Autodesk Inventor part; units mm, degrees
ref_plane "YZ Plane" through (0, 0, 0) normal (1, 0, 0) x (0, 1, 0)
ref_plane "XZ Plane" through (0, 0, 0) normal (0, 1, 0) x (-1, 0, 0)
ref_plane "XY Plane" through (0, 0, 0) normal (0, 0, 1) x (1, 0, 0)
sketch "Sketch1" plane through (0, 0, 0) normal (0, 1, 0) x (-1, 0, 0)
  line L0 (0, 0) -> (12.7, 0)
  line L1 (0, -129.6628) -> (0, 0)
  line L2 (0, -129.6628) -> (0, -142.3628)
  line L3 (0, -142.3628) -> (16.3017, -129.6628)
  line L4 (0, 0) -> (6.35, 0)
  line L5 (16.3017, -129.6628) -> (25.047, -123.1227)
  line L6 (6.35, 0) -> (18.1234, 0)
  line L7 (9.9069, 0) -> (25.047, -123.1227)
  circle A0 centre (4.9306, -5.8204) radius 4.445
  dimension "d10" = 8.89
sketch "Sketch2" plane through (0, 0, 0) normal (0, 1, 0) x (-1, 0, 0)
  point P0 (0, 0)
extrude "Extrusion1" add sketch "Sketch1" along normal blind 7.62 contours L0 L7 L5 L3 L2 L1 | A0
fillet "Fillet1" radius 25.4 1 edges at (-16.3017, 3.81, -129.6628)
sketch "Sketch3" plane through (0, 7.62, 0) normal (0, 1, 0) x (1, 0, 0)
  point P0 (0, 0)
sketch "Sketch4" plane through (0, 7.62, 0) normal (0, 1, 0) x (1, 0, 0)
  point P0 (0, 0)
sketch "Sketch5" plane through (0, 7.62, 0) normal (0, 1, 0) x (1, 0, 0)
  circle A0 centre (-5.6716, 10.0387) radius 4.5085
  point P0 (0, 0)
  dimension "d11" = 9.017
extrude "Extrusion2" cut sketch "Sketch5" against normal through all
fillet "Fillet2" radius 12.7 1 edges at (-25.047, 3.81, -123.1227)
fillet "Fillet3" radius 3.175 1 edges at (0, 3.81, -142.3628)
fillet "Fillet4" radius 3.175 12 edges at (-1.7812, 0, -138.7172) (-10.6152, 0, -134.0929) (-17.8257, 0, -128.5231) (-23.2248, 0, -122.3455) (-17.0275, 0, -57.9065) (0, 0, -67.9322) (-1.7812, 7.62, -138.7172) (-10.6152, 7.62, -134.0929) (-17.8257, 7.62, -128.5231) (-23.2248, 7.62, -122.3455) (-17.0275, 7.62, -57.9065) (0, 7.62, -67.9322)
properties part number "cock clamp" material "PC/ABS Plastic"
Input: part model. Units: mm. Frame: model coordinates. Round coordinates to 2 decimals unless told otherwise and drop trailing zeros. Loops run counter-clockwise (first coordinate to the right, second up) from the corner with the lowest first, then second, coordinate; pieces in that order, holes last. Notation, with made-up numbers: (89.5, -28.5) -> (117.5, -28.5) arc R31 cw to (117.5, -2.5) -> close; hole circle Ø6 at (79, 66). An arc over 180 degrees is marked (long way). Use one line per item in the form item = value. Start each with the question number.
Item 1: Material intervals for L1, parallel to Z at x = -5.5, y = 1.5; L2, parallel to Z at x = -7.5, y = 7.25; L3, parallel to X at y = 4, z = -97, sorted ascending. Write a range as from..to.
Item 2: Section query A-A on y = 5.75. Return the cut outline in (x, z) (1 decimal).
Item 3: Mould query, pull axis Z, two halves, no side actions, for faces 1 (the face through (-6.26, 3.86, -14.51)), 2 (the face through (-10.54, 3.8, -134.15)), 3 (the face through (-10, 7.62, -87)). Classes: pulls with the +Z half, pulls with the -Z half, needs draft (parallel to the pull), parting line crosses it, or undercut.
Item 4: Contact query for flat-ended pins moving along their axis: pin 1 Ø8 at (x, z) = (-5.67, -10.04) entering from +Y; pin 2 Ø4 at (y, z) = (3.5, -95.5) entering from -X; pin 3 Ø2 at (y, z) = (6.5, -90) entering from +X. Output: stop coordinate, or through.
Ans:
q1.L1 = -137.47..-14.54, -5.53..0
q1.L2 = -134.38..-14.16, -5.92..0
q1.L3 = -21.83..0
q2.outline = (-23.9, -115.8) arc R12.4 ccw to (-19, -127.3) -> (-16.3, -129.3) arc R25.7 cw to (-15.9, -129.6) -> (-5, -138.1) arc R2.9 ccw to (-0.3, -135.9) -> (-0.3, 0) -> (-9.6, 0) -> close; hole circle Ø9 at (-5.7, -10)
q3.face_1 = undercut
q3.face_2 = pulls with the -Z half
q3.face_3 = needs draft
q4.pin_1 = through
q4.pin_2 = -21.9
q4.pin_3 = -0.18
